Autodesk Inventor part; units mm, degrees
ref_plane "YZ Plane" through (0, 0, 0) normal (1, 0, 0) x (0, 1, 0)
ref_plane "XZ Plane" through (0, 0, 0) normal (0, 1, 0) x (-1, 0, 0)
ref_plane "XY Plane" through (0, 0, 0) normal (0, 0, 1) x (1, 0, 0)
sketch "Sketch1" plane through (0, 0, 0) normal (0, 0, 1) x (1, 0, 0)
  line L0 (33, -5.5) -> (-33, -5.5)
  line L1 (-33, -5.5) -> (-33, 5.5)
  line L2 (-33, 5.5) -> (33, 5.5)
  line L3 (33, 5.5) -> (33, -5.5)
  line L4 (33, -5.5) -> (-33, 5.5) construction
  line L5 (-33, -5.5) -> (33, 5.5) construction
  line L6 (-25, 3.5) -> (-79, 3.5)
  line L7 (-79, 3.5) -> (-79, -8.5)
  line L8 (-79, -8.5) -> (-25, -8.5)
  line L9 (-25, -8.5) -> (-25, 3.5)
  line L10 (0, 0) -> (0, 20.8366) construction
  line L11 (25, 3.5) -> (79, 3.5)
  line L12 (79, 3.5) -> (79, -8.5)
  line L13 (79, -8.5) -> (25, -8.5)
  line L14 (25, -8.5) -> (25, 3.5)
  point P0 (-25, -5.5)
  point P1 (25, -5.5)
  point P2 (33, 3.5)
  point P3 (-33, 3.5)
  dimension "d0" = 158
  dimension "d3" = 50
  dimension "d4" = 66
  dimension "d5" = 3
  dimension "d6" = 12
  dimension "d7" = 14
extrude "Extrusion1" add sketch "Sketch1" along normal mid plane 74
fillet "Fillet1" radius 3 2 edges at (25, -5.5, 0) (-25, -5.5, 0)
sketch "Sketch3" plane through (-79, 3.5, 37) normal (0, 1, 0) x (1, 0, 0)
  line L0 (46, 0) -> (0, 0)
  line L1 (0, 74) -> (0, 0)
  point P0 (79, 37)
  point P1 (12, 12)
  dimension "d11" = 12
  dimension "d12" = 12
hole "Hole1" at (-67, 3.5, 25) direction (0, -1, 0) diameter 10.106 end through all
pattern_linear "Rectangular Pattern1" count 2 spacing 50 along (0, 0, -1) count 2 spacing 134 along (1, 0, 0) of "Hole1"
fillet "Fillet2" radius 8 4 edges at (-79, -2.5, 37) (-79, -2.5, -37) (79, -2.5, -37) (79, -2.5, 37)
properties part number "01-base" material "Iron, Gray"
Model file for the job. Use its own axes, mm. A direction names the side the tool comes from. Give positions to 0.01 mm unless a question says otherwise; leave off trailing zeros. Loops run counter-clockwise (first coordinate to the right, second up) from the corner with the lowest first, then second, coordinate; pieces in that order, holes last. Notation, with made-up numbers: (85.5, 16) - (94.5, 16) arc R18 ccw to (94.5, 33) - close; hole circle Ø6 at (58, -20). An arc over 180 degrees is marked (long way). Use one line per item in the form item = value.
(1) Drop flat-ended pins along their axis: P1, Ø5, axis at x = 44, z = -14.5, coming from the +Y side; P2, Ø6, axis at x = -67, z = 25, coming from the -Y side; P3, Ø16, axis at x = 67, z = -25, coming from the -Y side; P4, Ø1, axis at y = 5, z = 8.5, coming from the +X side. Give the stop position or say it passes through.
Determined:
P1 = 3.5
P2 = through
P3 = -8.5
P4 = 33
(2) Cut at B-B (x = -67). Give the cut face in (y, z), then the cut area to 3 significant figures.
Determined:
outline = (-8.5, -37) - (3.5, -37) - (3.5, -30.05) - (-8.5, -30.05) - close; (-8.5, -19.95) - (3.5, -19.95) - (3.5, 19.95) - (-8.5, 19.95) - close; (-8.5, 30.05) - (3.5, 30.05) - (3.5, 37) - (-8.5, 37) - close
area = 645 mm^2
(3) Drill centre lines: L1, parallel to Z at x = 67, y = 1; L2, parallel to X at y = -5, z = 25; L3, parallel to X at y = 0.25, z = -26. Where is each one in solid material? Low to high.
Determined:
L1 = -37 to -30.05, -19.95 to 19.95, 30.05 to 37
L2 = -79 to -72.05, -61.95 to 61.95, 72.05 to 79
L3 = -79 to -71.95, -62.05 to 62.05, 71.95 to 79
(4) Cut at C-C (y = 0). Give the cut face in (x, z), then the cut area to 3 significant figures.
Determined:
outline = (-79, -29) arc R8 ccw to (-71, -37) - (71, -37) arc R8 ccw to (79, -29) - (79, 29) arc R8 ccw to (71, 37) - (-71, 37) arc R8 ccw to (-79, 29) - close; hole circle Ø10.11 at (-67, -25); hole circle Ø10.11 at (-67, 25); hole circle Ø10.11 at (67, -25); hole circle Ø10.11 at (67, 25)
area = 11,300 mm^2
(5) Cut at A-A (z = 25). Count the separate pieces of the cut face and the enclosed holes in it, then the cut area to 3 significant figures.
Determined:
separate_pieces = 3
enclosed_holes = 0
area = 1,640 mm^2
(6) 3-axis set-ups, long thin cutter, end or side, ignore diameter. For faces 5 (the face through (-56, 3.5, -1)), 6 (the face through (-1, -1, -37)), 7 (the face through (24.14, -6.4, 0.52)), 8 (the face through (56, 3.5, -1)): which of +Z, -Z, +X, -X, +Y, -Y reach the whole face in a straight line?
Determined:
face_5 = +Z, -Z, -X, +Y
face_6 = -Z, +X, -X, +Y, -Y
face_7 = +Z, -Z, -Y
face_8 = +Z, -Z, +X, +Y
(7) Pull direction X, two halves, no side cores. Call faces 1 (the face through (62.74, -2.58, -22.28)), 2 (the face through (-1, -1, 37)), 3 (the face through (76.594, -2.584, -34.719)), 4 (the face through (-76.719, -2.584, -34.594)): pulls with the +X half, pulls with the -X half, needs draft (parallel to the pull), parting line crosses it, or undercut.
Determined:
face_1 = undercut
face_2 = needs draft
face_3 = pulls with the +X half
face_4 = pulls with the -X half
